```python
from build123d import *

# Parameters (mm, degrees)
SKETCH_1_W          = 182
SKETCH_1_H          = 98
EXTRUDE_1_DEPTH     = 34.5
SHELL_1_T           = -2
SKETCH_2_R          = 32
CUT_EXTRUDE_1_DEPTH = 10
SKETCH_3_W          = 29.866450527
SKETCH_3_H          = 86.675289488
CUT_EXTRUDE_2_DEPTH = 10
FILLET_1_R          = 2
SKETCH_4_W          = 15
SKETCH_4_H          = 22
CUT_EXTRUDE_3_DEPTH = 10
FILLET_2_R          = 1
CHAMFER_1_SIZE      = 1


with BuildPart() as part:
    # 草图1 → 凸台-拉伸1 (new body)
    with BuildSketch(Plane(origin=(0, 0, 0), x_dir=(0, 0, -1), z_dir=(1, 0, 0))):
        with Locations((91, -49)):
            Rectangle(SKETCH_1_W, SKETCH_1_H)
    extrude(amount=EXTRUDE_1_DEPTH)

    # 抽壳1
    shell_1_openings = [part.faces().sort_by_distance(p)[0] for p in [
        (0, -49, -91),
    ]]
    offset(amount=SHELL_1_T, openings=shell_1_openings, kind=Kind.INTERSECTION)

    # 草图2 → 切除-拉伸1 (cut)
    with BuildSketch(Plane(origin=(34.5, 0, 0), x_dir=(0, 0, -1), z_dir=(1, 0, 0))):
        with Locations((38.698604665, -49)):
            Circle(SKETCH_2_R)
    extrude(amount=-CUT_EXTRUDE_1_DEPTH, mode=Mode.SUBTRACT)

    # 草图3 → 切除-拉伸2 (cut)
    with BuildSketch(Plane(origin=(0, 0, -182), x_dir=(-1, 0, 0), z_dir=(0, 0, -1))):
        with Locations((-14.933225264, -43.337644744)):
            Rectangle(SKETCH_3_W, SKETCH_3_H)
    extrude(amount=-CUT_EXTRUDE_2_DEPTH, mode=Mode.SUBTRACT)

    # 圆角1
    fillet_1_edges = [part.edges().sort_by_distance(p)[0] for p in [
        (34.5, 0, -91),
        (34.5, -49, 0),
        (17.25, 0, 0),
        (17.25, -98, 0),
        (34.5, -98, -91),
    ]]
    fillet(fillet_1_edges, radius=FILLET_1_R)

    # 草图4 → 切除-拉伸3 (cut)
    with BuildSketch(Plane(origin=(0, -98, 0), x_dir=(-1, 0, 0), z_dir=(0, -1, 0))):
        with Locations((-7.5, 21)):
            Rectangle(SKETCH_4_W, SKETCH_4_H)
    extrude(amount=-CUT_EXTRUDE_3_DEPTH, mode=Mode.SUBTRACT)

    # 圆角2
    fillet_2_edges = [part.edges().sort_by_distance(p)[0] for p in [
        (15, -97, -10),
        (15, -97, -32),
    ]]
    fillet(fillet_2_edges, radius=FILLET_2_R)

    # 倒角1
    chamfer_1_edges = [part.edges().sort_by_distance(p)[0] for p in [
        (34.5, -49, -6.698604665),
    ]]
    chamfer(chamfer_1_edges, length=CHAMFER_1_SIZE)


solid = part.part
```
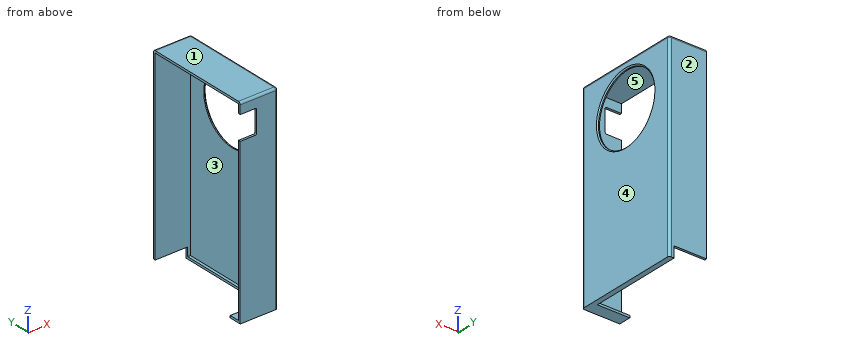
Build history of the part. All positions in model axes, mm. Face numbers are marked on the shaded views. A direction names the side the tool comes from. Give positions to 0.01 mm unless a question says otherwise; leave off trailing zeros. Loops run counter-clockwise (first coordinate to the right, second up) from the corner with the lowest first, then second, coordinate; pieces in that order, holes last. Notation, with made-up numbers: (-36.5, -7) -> (-12.5, -7) arc R26 ccw to (-12.5, 13) -> close; hole circle Ø5 at (-0.5, -2). An arc over 180 degrees is marked (long way). One line per question, with ' | ' between items.
Q1. Cut at B-B, the plane y = -49. Write the cut outline in (x, z), plus the area to 3 significant figures.
Filled sheet:
outline: (0, -2) -> (32.5, -2) -> (32.5, -6.7) -> (33.5, -6.7) -> (34.5, -5.7) -> (34.5, -2) arc R2 ccw to (32.5, 0) -> (0, 0) -> close; (29.87, -182) -> (34.5, -182) -> (34.5, -71.7) -> (33.5, -70.7) -> (32.5, -70.7) -> (32.5, -180) -> (29.87, -180) -> close | area: 304 mm²
Q2. Drop flat-ended pins along their axis: pin 1 (1.6 mm diameter, centred on y = -97, z = -21.5, fed in from -X); pin 2 (3 mm diameter, centred on y = -79, z = -46, fed in from +X); pin 3 (5 mm diameter, centred on y = -61.5, z = -175.5, fed in from -X). Give the stop position or say it passes through.
Filled sheet:
pin 1: stops at x = 15 | pin 2: stops at x = 33.88 | pin 3: stops at x = 32.5
Q3. Cut at C-C, the plane x = 17. Write the cut outline in (y, z).
Filled sheet:
outline: (-98, -182) -> (-86.68, -182) -> (-86.68, -180) -> (-96, -180) -> (-96, -2) -> (-2, -2) -> (-2, -172) -> (0, -172) -> (0, -2) arc R2 ccw to (-2, 0) -> (-96, 0) arc R2 ccw to (-98, -2) -> close
Q4. Pull direction Z, two halves, no side cores. Call the marked faces 1, 2 and 3: pulls with the +Z half, pulls with the -Z half, needs draft (parallel to the pull), parting line crosses it, or undercut.
Filled sheet:
face 1: pulls with the +Z half | face 2: needs draft | face 3: undercut
Q5. Cut at A-A, the plane x = 2. Write the cut outline in (y, z), plus the area to 3 significant figures.
Filled sheet:
outline: (-98, -182) -> (-86.68, -182) -> (-86.68, -180) -> (-96, -180) -> (-96, -32) -> (-98, -32) -> close; (-98, -10) -> (-96, -10) -> (-96, -2) -> (-2, -2) -> (-2, -172) -> (0, -172) -> (0, -2) arc R2 ccw to (-2, 0) -> (-96, 0) arc R2 ccw to (-98, -2) -> close | area: 869 mm²
Q6. Drill centre lines: line 1 along Y through (x, z) = (31, -94); line 2 along Z through (x, y) = (31, -70); line 3 along X through (y, z) = (-37, -167.5). Where is each one in solid material? Low to high. Write a range as [from, to].
Filled sheet:
line 1: y = [-98, -96], [-2, 0] | line 2: z = [-182, -180], [-2, 0] | line 3: x = [32.5, 34.5]
Q7. Tool access for the marked faces 4 and 5: list every direction of +Z, -Z, +X, -X, +Y, -Y with a clear straight run to the whole face (end or side of a thin tool).
Filled sheet:
face 4: +Z, -Z, +X, +Y, -Y | face 5: -X
Q8. Cut at D-D, the plane y = -91. Write the cut outline in (x, z), plus the area to 3 significant figures.
Filled sheet:
outline: (0, -182) -> (34.5, -182) -> (34.5, -2) arc R2 ccw to (32.5, 0) -> (0, 0) -> (0, -2) -> (32.5, -2) -> (32.5, -180) -> (0, -180) -> close | area: 493 mm²
